The model under review builds one solid part; all positions refer to its coordinate system, in mm. A direction names the side the tool comes from. Round coordinates to 2 decimals unless told otherwise and drop trailing zeros. Loops run counter-clockwise (first coordinate to the right, second up) from the corner with the lowest first, then second, coordinate; pieces in that order, holes last. Notation, with made-up numbers: (9, 56.5) - (56, 56.5) arc R23 cw to (56, 93.5) - close; hole circle Ø6 at (-39, -4.75). An arc over 180 degrees is marked (long way). Answer as CSV lines item,"result".
Autodesk Inventor part; units mm, degrees
ref_plane "YZ Plane" through (0, 0, 0) normal (1, 0, 0) x (0, 1, 0)
ref_plane "XZ Plane" through (0, 0, 0) normal (0, 1, 0) x (-1, 0, 0)
ref_plane "XY Plane" through (0, 0, 0) normal (0, 0, 1) x (1, 0, 0)
sketch "Sketch1" plane through (0, 0, 0) normal (0, 1, 0) x (-1, 0, 0)
  line L0 (15, 13) -> (-15, 13)
  line L1 (-15, 13) -> (-15, -13)
  line L2 (-15, -13) -> (15, -13)
  line L3 (15, -13) -> (15, 13)
  line L4 (15, 13) -> (-15, -13) construction
  line L5 (-15, 13) -> (15, -13) construction
  circle A0 centre (-14, 4) radius 0.5
  circle A1 centre (14, 4) radius 0.5
  circle A2 centre (14, -4) radius 0.5
  circle A3 centre (-14, -4) radius 0.5
  line L6 (-11, 17) -> (-19, 17)
  line L7 (-19, 17) -> (-19, 9)
  line L8 (-19, 9) -> (-11, 9)
  line L9 (-11, 9) -> (-11, 17)
  line L10 (-11, 17) -> (-19, 9) construction
  line L11 (-19, 17) -> (-11, 9) construction
  line L12 (19, 9) -> (11, 9)
  line L13 (11, 9) -> (11, 17)
  line L14 (11, 17) -> (19, 17)
  line L15 (19, 17) -> (19, 9)
  line L16 (19, 9) -> (11, 17) construction
  line L17 (11, 9) -> (19, 17) construction
  line L18 (19, -17) -> (11, -17)
  line L19 (11, -17) -> (11, -9)
  line L20 (11, -9) -> (19, -9)
  line L21 (19, -9) -> (19, -17)
  line L22 (19, -17) -> (11, -9) construction
  line L23 (11, -17) -> (19, -9) construction
  line L24 (-11, -9) -> (-19, -9)
  line L25 (-19, -9) -> (-19, -17)
  line L26 (-19, -17) -> (-11, -17)
  line L27 (-11, -17) -> (-11, -9)
  line L28 (-11, -9) -> (-19, -17) construction
  line L29 (-19, -9) -> (-11, -17) construction
  point P0 (0, 0)
  point P1 (11, 13)
  point P2 (15, 9)
  point P3 (15, -9)
  point P4 (11, -13)
  point P5 (-11, -13)
  point P6 (-15, -9)
  point P7 (-15, 9)
  point P8 (-11, 13)
  dimension "d0" = 30
  dimension "d1" = 26
  dimension "d4" = 1
  dimension "d5" = 9
  dimension "d6" = 1
  dimension "d7" = 1
  dimension "d8" = 1
  dimension "d9" = 1
  dimension "d10" = 1
  dimension "d11" = 9
  dimension "d12" = 1
  dimension "d13" = 9
  dimension "d14" = 9
  dimension "d15" = 1
  dimension "d24" = 8
  dimension "d25" = 8
  dimension "d26" = 8
  dimension "d27" = 8
  dimension "d28" = 8
  dimension "d29" = 8
  dimension "d30" = 8
  dimension "d31" = 8
extrude "Extrusion1" add sketch "Sketch1" along normal blind 1
sketch "Sketch3" plane through (0, 1, 0) normal (0, 1, 0) x (1, 0, 0)
  line L0 (15, -9) -> (15, 9)
  line L1 (15, 9) -> (19, 9)
  line L2 (19, 9) -> (19, 17)
  line L3 (19, 17) -> (11, 17)
  line L4 (11, 17) -> (11, 13)
  line L5 (11, 13) -> (-11, 13)
  line L6 (-11, 13) -> (-11, 17)
  line L7 (-11, 17) -> (-19, 17)
  line L8 (-19, 17) -> (-19, 9)
  line L9 (-19, 9) -> (-15, 9)
  line L10 (-15, 9) -> (-15, -9)
  line L11 (-15, -9) -> (-19, -9)
  line L12 (-19, -9) -> (-19, -17)
  line L13 (-19, -17) -> (-11, -17)
  line L14 (-11, -17) -> (-11, -13)
  line L15 (-11, -13) -> (11, -13)
  line L16 (11, -13) -> (11, -17)
  line L17 (11, -17) -> (19, -17)
  line L18 (19, -17) -> (19, -9)
  line L19 (19, -9) -> (15, -9)
  circle A0 centre (14, -4) radius 0.5
  circle A1 centre (-14, -4) radius 0.5
  circle A2 centre (-14, 4) radius 0.5
  circle A3 centre (14, 4) radius 0.5
  circle A4 centre (-7.5, 0) radius 0.5
  circle A5 centre (7.5, 0) radius 0.5
  point P0 (0, 0)
  dimension "d32" = 1
  dimension "d33" = 1
  dimension "d34" = 7.5
  dimension "d35" = 7.5
extrude "Extrusion2" add sketch "Sketch3" along normal blind 3.5 contours A4 | A5
sketch "Sketch4" plane through (0, 0, 0) normal (0, -1, 0) x (1, 0, 0)
  line L0 (15, 9) -> (15, -9)
  line L1 (19, 9) -> (15, 9)
  line L2 (19, 17) -> (19, 9)
  line L3 (11, 17) -> (19, 17)
  line L4 (11, 13) -> (11, 17)
  line L5 (-11, 13) -> (11, 13)
  line L6 (-11, 17) -> (-11, 13)
  line L7 (-19, 17) -> (-11, 17)
  line L8 (-19, 9) -> (-19, 17)
  line L9 (-15, 9) -> (-19, 9)
  line L10 (-15, -9) -> (-15, 9)
  line L11 (-19, -9) -> (-15, -9)
  line L12 (-19, -17) -> (-19, -9)
  line L13 (-11, -17) -> (-19, -17)
  line L14 (-11, -13) -> (-11, -17)
  line L15 (11, -13) -> (-11, -13)
  line L16 (11, -17) -> (11, -13)
  line L17 (19, -17) -> (11, -17)
  line L18 (19, -9) -> (19, -17)
  line L19 (15, -9) -> (19, -9)
  circle A0 centre (14, 4) radius 0.5
  circle A1 centre (-14, 4) radius 0.5
  circle A2 centre (-14, -4) radius 0.5
  circle A3 centre (14, -4) radius 0.5
  circle A4 centre (-7.5, 0) radius 0.5
  circle A5 centre (7.5, 0) radius 0.5
  point P0 (0, 0)
extrude "Extrusion3" cut sketch "Sketch4" against normal blind 0.5 contours A4 | A5
equation "\"d24\" = d25"
equation "\"d26\" = d25"
equation "\"d27\" = d25"
equation "\"d28\" = d25"
equation "\"d29\" = d25"
equation "\"d30\" = d25"
equation "\"d31\" = d25"
properties part number "base"
1. Take a section at D-D (x = 7.5). State the section outline as (y, z) points, plus the area to 3 significant figures.
Numbers:
outline,"(0, -13) - (1, -13) - (1, -0.5) - (4.5, -0.5) - (4.5, 0.5) - (1, 0.5) - (1, 13) - (0, 13) - (0, 0.5) - (0.5, 0.5) - (0.5, -0.5) - (0, -0.5) - close"
area,"29.0 mm²"
2. Take a section at C-C (z = -13.5). State the section outline as (x, y) points.
Numbers:
outline,"(-19, 0) - (-11, 0) - (-11, 1) - (-19, 1) - close; (11, 0) - (19, 0) - (19, 1) - (11, 1) - close"
3. Clearance check with flat-ended pins moving along their axes: pin 1 (1 mm diameter, centred on y = 2.5, z = 12.5, fed in from -X); pin 2 (0.8 mm diameter, centred on y = 0.5, z = 3.5, fed in from +X); pin 3 (12 mm diameter, centred on x = 0, z = -1.5, fed in from +Y); pin 4 (0.8 mm diameter, centred on x = 4.5, y = 0.5, fed in from +Z). State where each tip first meets the part, or that it passes through.
Numbers:
pin 1,"passes through"
pin 2,"stops at x = 15"
pin 3,"stops at y = 1"
pin 4,"stops at z = 13"
4. Take a section at A-A (x = 14). State the section outline as (y, z) points.
Numbers:
outline,"(0, -17) - (1, -17) - (1, -4.5) - (0, -4.5) - close; (0, -3.5) - (1, -3.5) - (1, 3.5) - (0, 3.5) - close; (0, 4.5) - (1, 4.5) - (1, 17) - (0, 17) - close"
5. Draft analysis for pull direction Z (two halves, no side actions). For faces 1 (the face through (-14.9, 0.5, 17)), 2 (the face through (19, 0.5, 13.1)), 3 (the face through (-15, 0.5, -0.1)), state which applies: +Z half, -Z half, draft (parallel to the pull), parting line (faces both ways), or undercut.
Numbers:
face 1,"+Z half"
face 2,"draft"
face 3,"undercut"
6. Wall thickness on probe 1 along Z at (x, y) = (-14, 0.3); probe 2 along Z at (x, y) = (-7.5, 0.3); probe 3 along X at (y, z) = (1.2, 0): over which ranges is each line inside the solid? List them lowest first.
Numbers:
probe 1,"z = -17 to -4.5, -3.5 to 3.5, 4.5 to 17"
probe 2,"z = -13 to -0.5, 0.5 to 13"
probe 3,"x = -8 to -7, 7 to 8"
7. Tool access review of faces 4 (the face through (-7.023, 0.246, 0.15)), 5 (the face through (-0.2, 0.5, 13)), 6 (the face through (-17, 0.5, -9)): name each direction out of +Z, -Z, +X, -X, +Y, -Y from which nothing blocks a thin tool from reaching the whole face with its end or side.
Numbers:
face 4,"-Y"
face 5,"+Z, +Y, -Y"
face 6,"-X, +Y, -Y"
8. Take a section at B-B (z = -4). State the section outline as (x, y) points, plus the area to 3 significant figures.
Numbers:
outline,"(-15, 0) - (-14.5, 0) - (-14.5, 1) - (-15, 1) - close; (-13.5, 0) - (13.5, 0) - (13.5, 1) - (-13.5, 1) - close; (14.5, 0) - (15, 0) - (15, 1) - (14.5, 1) - close"
area,"28.0 mm²"
